```python
from build123d import *

# Parameters (mm, degrees)
SKETCH1_W           = 76.2
SKETCH1_H           = 76.2
SKETCH1_W_2         = 12.7
SKETCH1_H_2         = 6.35
SKETCH1_W_3         = 6.35
SKETCH1_H_3         = 12.7
BOSS_EXTRUDE1_DEPTH = 12.7


with BuildPart() as part:
    # Sketch1 → Boss-Extrude1 (new body)
    with BuildSketch(Plane(origin=(0, 0, 0), x_dir=(1, 0, 0), z_dir=(0, 1, 0))):
        Rectangle(SKETCH1_W, SKETCH1_H)
        with Locations((-25.4, 0)):
            Rectangle(SKETCH1_W_2, SKETCH1_H_2, mode=Mode.SUBTRACT)
        with Locations((-25.4, 12.7)):
            Rectangle(SKETCH1_W_2, SKETCH1_H_2, mode=Mode.SUBTRACT)
        with Locations((-25.4, -12.7)):
            Rectangle(SKETCH1_W_2, SKETCH1_H_2, mode=Mode.SUBTRACT)
        with Locations((-25.4, -25.4)):
            Rectangle(SKETCH1_W_2, SKETCH1_H_2, mode=Mode.SUBTRACT)
        with Locations((3.719341062, 25.4)):
            Rectangle(SKETCH1_W_3, SKETCH1_H_3, mode=Mode.SUBTRACT)
        with Locations((-8.980658938, 25.4)):
            Rectangle(SKETCH1_W_3, SKETCH1_H_3, mode=Mode.SUBTRACT)
        with Locations((16.419341062, 25.4)):
            Rectangle(SKETCH1_W_3, SKETCH1_H_3, mode=Mode.SUBTRACT)
        with Locations((29.119341062, 25.4)):
            Rectangle(SKETCH1_W_3, SKETCH1_H_3, mode=Mode.SUBTRACT)
    extrude(amount=BOSS_EXTRUDE1_DEPTH)


solid = part.part
```
Geometry check sheet. Reference: the model listing, model coordinates, mm. Coordinates: 2 decimals unless noted, no trailing zeros. Loops run counter-clockwise (first coordinate to the right, second up) from the corner with the lowest first, then second, coordinate; pieces in that order, holes last.
Item 1: Sectioned sample at A-A, the plane x = -21. Record the boundary of the cut face in (y, z) (3 decimals), then the cut area to 3 significant figures.
Item 2: Thickness scan on line 1 (Z direction, x = -28.5, y = 5.25) (3 decimals); line 2 (X direction, y = 9.5, z = -30.5); line 3 (Z direction, x = 32, y = 11.75). Record the ranges inside material, lowest first.
Item 3: Sectioned sample at C-C, the plane y = 10.5. Count the separate pieces of the cut face and the enclosed holes in it, then the cut area to 3 significant figures.
Item 4: Release check for a two-part mould opening along Z. For faces 1 (the face through (-19.05, 6, 0)), 2 (the face through (-5.806, 6, -25)) record: released by +Z, released by -Z, zero draft, split by the parting line, or undercut.
Item 5: Sectioned sample at B-B, the plane z = 12. Record the boundary of the cut face in (x, y).
Check result:
1. outline: (0, -38.1) - (12.7, -38.1) - (12.7, -15.875) - (0, -15.875) - close; (0, -9.525) - (12.7, -9.525) - (12.7, -3.175) - (0, -3.175) - close; (0, 3.175) - (12.7, 3.175) - (12.7, 9.525) - (0, 9.525) - close; (0, 15.875) - (12.7, 15.875) - (12.7, 22.225) - (0, 22.225) - close; (0, 28.575) - (12.7, 28.575) - (12.7, 38.1) - (0, 38.1) - close
1. area: 645 mm2
2. line 1: z = -38.1 to -15.875, -9.525 to -3.175, 3.175 to 9.525, 15.875 to 22.225, 28.575 to 38.1
2. line 2: x = -38.1 to -12.16, -5.81 to 0.54, 6.89 to 13.24, 19.59 to 25.94, 32.29 to 38.1
2. line 3: z = -38.1 to -31.75, -19.05 to 38.1
3. separate pieces: 1
3. enclosed holes: 8
3. area: 5,160 mm2
4. face 1: undercut
4. face 2: undercut
5. outline: (-38.1, 0) - (-31.75, 0) - (-31.75, 12.7) - (-38.1, 12.7) - close; (-19.05, 0) - (38.1, 0) - (38.1, 12.7) - (-19.05, 12.7) - close
